Could you check a few things on this model? Use its own coordinates, in mm. A direction names the side the tool comes from. Coordinates: 2 decimals unless noted, no trailing zeros. Order: outer loops, then holes, each group sorted by start corner. A loop starts at its lowest first (then second) coordinate and runs counter-clockwise, first axis right, second up. Notation, with made-up numbers: (64, 24) - (96, 24) arc R27 ccw to (96, 55) - close; hole circle Ø5 at (6.5, 57). An arc over 180 degrees is marked (long way). One line per item, written item: value.
from build123d import *

# Parameters (mm, degrees)
F1_DEPTH  = 5.08
F2_R      = 40
F2_R_2    = 46.5
F2_R_3    = 1.27
F3_DEPTH  = 25.4
F4_W      = 115.731926
F4_H      = 4.953
F5_DEPTH  = 5.081
F6_R      = 7.8867
F7_DEPTH  = 2.54
F8_R      = 1.27
F9_DEPTH  = 2.541
F10_W     = 2.54
F10_H     = 0.254
F11_DEPTH = 5.081


with BuildPart() as f1:
    # F0 (on Top) → F1 (new body)
    with BuildSketch(Plane.XY):
        with BuildLine():
            Line((-79.922598, 113.03), (-137.84815, 12.7))
            ThreePointArc((-137.84815, 12.7), (-141.251105, 0), (-137.84815, -12.7))
            Line((-137.84815, -12.7), (-79.922598, -113.03))
            ThreePointArc((-79.922598, -113.03), (-70.625553, -122.327045), (-57.925553, -125.73))
            Line((-57.925553, -125.73), (57.925553, -125.73))
            ThreePointArc((57.925553, -125.73), (70.625553, -122.327045), (79.922598, -113.03))
            Line((79.922598, -113.03), (137.84815, -12.7))
            ThreePointArc((137.84815, -12.7), (141.251105, 0), (137.84815, 12.7))
            Line((137.84815, 12.7), (79.922598, 113.03))
            ThreePointArc((79.922598, 113.03), (70.625553, 122.327045), (57.925553, 125.73))
            Line((57.925553, 125.73), (-57.925553, 125.73))
            ThreePointArc((-57.925553, 125.73), (-70.625553, 122.327045), (-79.922598, 113.03))
        make_face()
    extrude(amount=F1_DEPTH)

    # F2 (on face) → F3 (cut)
    with BuildSketch(Plane.XY.offset(5.08)):
        with Locations((0, 62.23)):
            Circle(F2_R)
        with Locations((0, -55.88)):
            Circle(F2_R_2)
        with Locations((57.15, -55.88)):
            Circle(F2_R_3)
        with Locations((30.284886, -7.414051)):
            Circle(F2_R_3)
        with Locations((30.284886, -104.345949)):
            Circle(F2_R_3)
        with Locations((-30.284886, -7.414051)):
            Circle(F2_R_3)
        with Locations((-30.284886, -104.345949)):
            Circle(F2_R_3)
        with Locations((-57.15, -55.88)):
            Circle(F2_R_3)
        with Locations((-32.880465, 95.110465)):
            Circle(F2_R_3)
        with Locations((-32.880465, 29.349535)):
            Circle(F2_R_3)
        with Locations((32.880465, 29.349535)):
            Circle(F2_R_3)
        with Locations((32.880465, 95.110465)):
            Circle(F2_R_3)
    extrude(amount=-F3_DEPTH, mode=Mode.SUBTRACT)

    # F4 (on face) → F5 (cut, through all)
    with BuildSketch(Plane.XY.offset(5.08)):
        Polygon((-135.03893, -11.215713), (-77.172967, -111.4425), (-72.883543, -108.966), (-130.749506, -8.739213), align=None)
        Polygon((-77.232557, 111.339287), (-135.09852, 11.1125), (-130.809096, 8.636), (-72.943133, 108.862787), align=None)
        with Locations((-0.05959, 120.0785)):
            Rectangle(F4_W, F4_H)
        Polygon((135.03893, 11.215713), (77.172967, 111.4425), (72.883543, 108.966), (130.749506, 8.739213), align=None)
        Polygon((77.232557, -111.339287), (135.09852, -11.1125), (130.809096, -8.636), (72.943133, -108.862787), align=None)
        with Locations((0.05959, -120.0785)):
            Rectangle(F4_W, F4_H)
    extrude(amount=-F5_DEPTH, mode=Mode.SUBTRACT)

    # F6 (on face) → F7 (cut)
    with BuildSketch(Plane.XY.offset(5.08)):
        with Locations((-61.343372, 106.202414)):
            Circle(F6_R)
        with Locations((61.302302, 106.226125)):
            Circle(F6_R)
        with Locations((122.645674, 0.023711)):
            Circle(F6_R)
        with Locations((61.343372, -106.202414)):
            Circle(F6_R)
        with Locations((-61.302302, -106.226125)):
            Circle(F6_R)
        with Locations((-122.645674, -0.023711)):
            Circle(F6_R)
    extrude(amount=-F7_DEPTH, mode=Mode.SUBTRACT)

    # F8 (on face) → F9 (cut, through all)
    with BuildSketch(Plane.XY.offset(2.54)):
        with Locations((-61.343372, 106.202414)):
            Circle(F8_R)
        with Locations((61.302302, 106.226125)):
            Circle(F8_R)
        with Locations((-61.302302, -106.226125)):
            Circle(F8_R)
        with Locations((61.343372, -106.202414)):
            Circle(F8_R)
        with Locations((122.645674, 0.023711)):
            Circle(F8_R)
        with Locations((-122.645674, -0.023711)):
            Circle(F8_R)
    extrude(amount=-F9_DEPTH, mode=Mode.SUBTRACT)

    # F10 (on face) → F11 (cut, through all)
    with BuildSketch(Plane.XY.offset(5.08)):
        with Locations((-9.525, -125.603)):
            Rectangle(F10_W, F10_H)
        with Locations((9.58459, -125.603)):
            Rectangle(F10_W, F10_H)
    extrude(amount=-F11_DEPTH, mode=Mode.SUBTRACT)


solid = f1.part
Item 1: I want a section at D-D on y = -80.5. Please give me the cut outline in (x, z), then the cut area to 3 significant figures.
Conclusion:
outline: (-98.7, 0) - (-95.04, 0) - (-95.04, 5.08) - (-98.7, 5.08) - close; (-89.32, 0) - (-39.45, 0) - (-39.45, 5.08) - (-89.32, 5.08) - close; (39.45, 0) - (89.32, 0) - (89.32, 5.08) - (39.45, 5.08) - close; (95.04, 0) - (98.7, 0) - (98.7, 5.08) - (95.04, 5.08) - close
area: 544 mm²
Item 2: I want a section at B-B on x = -108. Please give me the cut outline in (y, z).
Conclusion:
outline: (-64.4, 0) - (-58.05, 0) - (-58.05, 5.08) - (-64.4, 5.08) - close; (-48.14, 0) - (48.14, 0) - (48.14, 5.08) - (-48.14, 5.08) - close; (58.05, 0) - (64.4, 0) - (64.4, 5.08) - (58.05, 5.08) - close
Item 3: If I drill on probe 1 along Y at (x, z) = (1, 1.65) (1 decimal); probe 2 along Y at (x, z) = (48, 3.65) (3 decimals); probe 3 along X at (y, z) = (0, 2.65), over which ranges is the centre line in solid material (lowest first)?
Conclusion:
probe 1: -125.7 to -122.6, -117.6 to -102.4, -9.4 to 22.2, 102.2 to 117.6, 122.6 to 125.7
probe 2: -125.73 to -122.555, -117.602 to 117.602, 122.555 to 125.73
probe 3: -141.25 to -130.53, -114.76 to 114.76, 130.53 to 141.25
Item 4: Thinking about a two-plate mould opening in X: for faces 1 (the face through (102.28, -58.05, 2.58)), 2 (the face through (-2, 2, 5.08)), 3 (the face through (109.291, 62.163, 2.504)), which applies, pulls with the +X half, pulls with the -X half, needs draft (parallel to the pull), parting line crosses it, or undercut?
Conclusion:
face 1: undercut
face 2: needs draft
face 3: pulls with the +X half
Item 5: I want a section at A-A on y = 53.5. Please give me the cut outline in (x, z).
Conclusion:
outline: (-114.29, 0) - (-110.63, 0) - (-110.63, 5.08) - (-114.29, 5.08) - close; (-104.91, 0) - (-39.04, 0) - (-39.04, 5.08) - (-104.91, 5.08) - close; (39.04, 0) - (104.91, 0) - (104.91, 5.08) - (39.04, 5.08) - close; (110.63, 0) - (114.29, 0) - (114.29, 5.08) - (110.63, 5.08) - close
Item 6: I'm going to push flat-ended pins straight in: pin 1 Ø20.5 at (x, y) = (61.3, 106.23) entering from -Z; pin 2 Ø3 at (y, z) = (14, 1.5) entering from -X; pin 3 Ø2 at (y, z) = (-63.5, 2.5) entering from +X; pin 4 Ø1.3 at (x, z) = (-9.5, 4) entering from -Y. Where does each tip first touch, or does it pass through?
Conclusion:
pin 1: z = 0
pin 2: x = -137.96
pin 3: x = 109.1
pin 4: y = -125.48
Item 7: I want a section at C-C on x = -2. Please give me the cut outline in (y, z) (3 decimals).
Conclusion:
outline: (-125.73, 0) - (-122.555, 0) - (-122.555, 5.08) - (-125.73, 5.08) - close; (-117.602, 0) - (-102.337, 0) - (-102.337, 5.08) - (-117.602, 5.08) - close; (-9.423, 0) - (22.28, 0) - (22.28, 5.08) - (-9.423, 5.08) - close; (102.18, 0) - (117.602, 0) - (117.602, 5.08) - (102.18, 5.08) - close; (122.555, 0) - (125.73, 0) - (125.73, 5.08) - (122.555, 5.08) - close
Item 8: For faces 4 (the face through (105.76, -61.93, 2.58)), 5 (the face through (-128.904, -4.823, 3.828)), 6 (the face through (-70.5, 122.4, 2.5)), which set-ups out of +Z, -Z, +X, -X, +Y, -Y let a thin tool reach every point of the face, with its end or its side?
Conclusion:
face 4: +Z, -Z
face 5: +Z
face 6: +Z, -Z, -X, +Y
